Geometry check sheet. Reference: the model listing, model coordinates, mm. Face numbers are marked on the shaded views. A direction names the side the tool comes from. Give positions to 0.01 mm unless a question says otherwise; leave off trailing zeros. Write each loop counter-clockwise with the first axis right and the second up, starting at its lowest first coordinate (ties: lowest second). Pieces come first, ordered by that corner, then holes.
(1) Cross-section at A-A (y = -73.5). Record the boundary of the cut face in (x, z).
(2) Mould release check, pull along Z, two halves, no side actions. Record for the marked faces 5, 6, 7 and 8: +Z half, -Z half, draft (parallel to the pull), parting line (faces both ways), or undercut.
(3) Cross-section at D-D (x = -15). Record the boundary of the cut face in (y, z).
(4) Thickness scan on line 1 along X through (y, z) = (38.5, 31); line 2 along X through (y, z) = (-43.5, 8); line 3 along X through (y, z) = (-17, 9.5). Record the ranges inside material, lowest first.
(5) Depth check by flat-ended pin: P1, Ø8.5, axis at y = -48.5, z = 21.5, coming from the -X side; P2, Ø1, axis at y = 0.5, z = 5.5, coming from the -X side; P3, Ø0.9, axis at y = 38.5, z = 38.5, coming from the -X side. Enter the tip coordinate at first touch or a pass-through.
(6) Cross-section at B-B (x = 38). Record the boundary of the cut face in (y, z).
(7) Tool access check on the marked faces 1, 2, 3 and 4. Record the directions out of +Z, -Z, +X, -X, +Y, -Y that give a thin tool (end or side, any length) a straight path to the whole face; none if there is none.
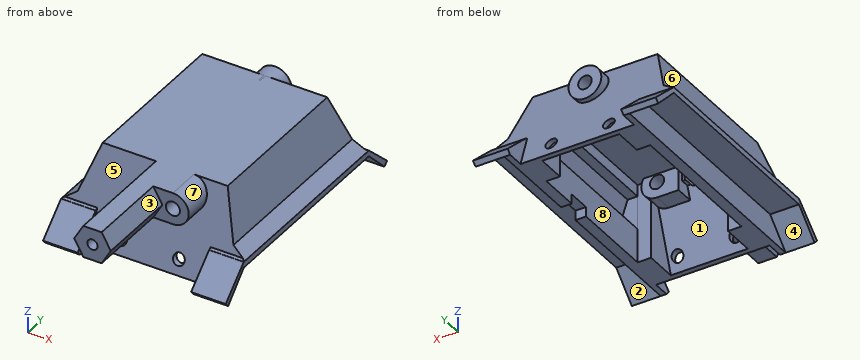
```python
from build123d import *

# Parameters (mm, degrees)
SKETCH_W             = 65
SKETCH_H             = 83
PAD_DEPTH            = 45
SKETCH001_W          = 83
SKETCH001_H          = 32
PAD001_DEPTH         = 15
PAD002_DEPTH         = 15
POCKET_DEPTH         = 403.6691065481
POCKET001_DEPTH      = 500
POCKET001_DEPTH_BACK = 100
PAD003_DEPTH         = 16
SKETCH007_W          = 3
SKETCH007_H          = 135.5960614908
PAD004_DEPTH         = 16
POCKET002_DEPTH      = 414.7315387876
POCKET003_DEPTH      = 5
SKETCH008_W          = 54
SKETCH008_H          = 76
POCKET004_DEPTH      = 35
PAD005_DEPTH         = 65
CHAMFER_SIZE         = 5.3
CHAMFER001_SIZE      = 5.3
CHAMFER002_SIZE      = 0.8999
CHAMFER003_SIZE      = 0.899
CHAMFER004_SIZE      = 0.8999
CHAMFER005_SIZE      = 0.8999
POCKET005_DEPTH      = 80.0010001
POCKET006_DEPTH      = 80.0010001
POCKET007_DEPTH      = 10000
POCKET007_DEPTH_BACK = 100
POCKET008_DEPTH      = 95.001
SKETCH012_W          = 5.5
SKETCH012_H          = 12
POCKET009_DEPTH      = 5
POCKET010_DEPTH      = 20
POCKET010_DEPTH_BACK = 20
POCKET011_DEPTH      = 6
SKETCH014_R          = 8.518625
PAD006_DEPTH         = 13
SKETCH015_R          = 3.5
POCKET012_DEPTH      = 15
SKETCH016_R          = 0.75
POCKET013_DEPTH      = 40
SKETCH018_W          = 5.5
SKETCH018_H          = 12
POCKET014_DEPTH      = 5
POCKET014_FACE131_W  = 12
POCKET014_FACE131_H  = 5.5
PAD007_DEPTH         = 5
POCKET015_DEPTH      = 38.88
POCKET015_DEPTH_BACK = 37
SKETCH020_R          = 3
POCKET016_DEPTH      = 173.1015589479
SKETCH021_R          = 2.7
POCKET017_DEPTH      = 70
SKETCH022_R          = 3.6
PAD008_DEPTH         = 25
SKETCH023_R          = 3.660532
POCKET018_DEPTH      = 25
SKETCH024_W          = 7
SKETCH024_H          = 6.387993
POCKET019_DEPTH      = 40


with BuildPart() as part:
    # Sketch → Pad (new body)
    with BuildSketch(Plane.XY):
        Rectangle(SKETCH_W, SKETCH_H)
    extrude(amount=PAD_DEPTH)

    # Sketch001 (on Face4 of Pad) → Pad001 (join)
    with BuildSketch(Plane(origin=(-32.5, 0, 0), x_dir=(0, -1, 0), z_dir=(-1, 0, 0))):
        with Locations((0, 29)):
            Rectangle(SKETCH001_W, SKETCH001_H)
    pad001 = extrude(amount=PAD001_DEPTH)

    # Mirrored: Pad001 across YZ
    add(pad001.mirror(Plane.YZ))

    # Sketch002 (on Face4 of Mirrored) → Pad002 (join)
    with BuildSketch(Plane.XZ.offset(41.5)):
        Polygon((-47.5, 45), (47.5, 45), (47.5, 13), (32.5, 13), (32.5, 0), (-32.5, 0), (-32.5, 13), (-47.5, 13), align=None)
    pad002 = extrude(amount=PAD002_DEPTH)

    # Mirrored001: Pad002 across XZ
    add(pad002.mirror(Plane.XZ))

    # Sketch003 (on Face13 of Mirrored001) → Pocket (cut, through all)
    with BuildSketch(Plane(origin=(-47.5, 0, 0), x_dir=(0, -1, 0), z_dir=(-1, 0, 0))):
        Polygon((41.5, 45), (56.5, 0), (69.973511, 50.863071), align=None)
    pocket = extrude(amount=-POCKET_DEPTH, mode=Mode.SUBTRACT)

    # Mirrored002: Pocket across XZ
    add(pocket.mirror(Plane.XZ), mode=Mode.SUBTRACT)

    # Sketch004 → Pocket001 (cut, two sides)
    with BuildSketch(Plane.XZ) as pocket001_sk:
        Polygon((-32.5, 45), (-47.5, 0), (-68.972275, 31.059837), (-58.790833, 51.045628), align=None)
    pocket001 = extrude(amount=-POCKET001_DEPTH, mode=Mode.SUBTRACT) + extrude(pocket001_sk.sketch, amount=POCKET001_DEPTH_BACK, mode=Mode.SUBTRACT)

    # Mirrored003: Pocket001 across YZ
    add(pocket001.mirror(Plane.YZ), mode=Mode.SUBTRACT)

    # Sketch006 (on DatumPlane) → Pad003 (join)
    with BuildSketch(Plane(origin=(-47.5, 0, 4), x_dir=(0, -1, 0), z_dir=(-1, 0, 0))):
        Polygon((-68.401131891, -2.9951612268), (-52.1666666667, 12), (52.1666666667, 12), (67.1949295998, -1.7895363668), (65.1666666666, -4), (52.1666666667, 9), (-52.1666666667, 9), (-66.3655953138, -5.1989286472), align=None)
    pad003 = extrude(amount=-PAD003_DEPTH)

    # Sketch007 (on Face8 of Pad003) → Pad004 (join)
    with BuildSketch(Plane(origin=(0, 0, 0), x_dir=(1, 0, 0), z_dir=(0, 0, -1))):
        with Locations((-31, -0.6031011456)):
            Rectangle(SKETCH007_W, SKETCH007_H)
    pad004 = extrude(amount=-PAD004_DEPTH)

    # Pad004 Face41 → Pocket002 (cut, through all)
    with BuildSketch(Plane(origin=(-32.5, 62.9896434829, 11.0016129244), x_dir=(0, 1, 0), z_dir=(-1, 0, 0))):
        Polygon((5.4114884081, -4.9983870756), (5.4114884081, 9.9967741512), (-10.8229768162, -4.9983870756), align=None)
    pocket002 = extrude(amount=-POCKET002_DEPTH, mode=Mode.SUBTRACT)

    # Pocket002 Face27 → Pocket003 (cut)
    with BuildSketch(Plane(origin=(-32.5, -62.1855086221, 11.4034878777), x_dir=(0, 1, 0), z_dir=(-1, 0, 0))):
        Polygon((10.0188419554, -4.5965121223), (-5.0094209777, 9.1930242445), (-5.0094209777, -4.5965121223), align=None)
    pocket003 = extrude(amount=-POCKET003_DEPTH, mode=Mode.SUBTRACT)

    # Mirrored004: Pad003 across YZ
    add(pad003.mirror(Plane.YZ))

    # Mirrored005: Pad004 across YZ
    add(pad004.mirror(Plane.YZ))

    # Mirrored006: Pocket002 across YZ
    add(pocket002.mirror(Plane.YZ), mode=Mode.SUBTRACT)

    # Mirrored007: Pocket003 across YZ
    add(pocket003.mirror(Plane.YZ), mode=Mode.SUBTRACT)

    # Sketch008 (on Face8 of Mirrored007) → Pocket004 (cut)
    with BuildSketch(Plane(origin=(0, 0, 0), x_dir=(1, 0, 0), z_dir=(0, 0, -1))):
        with Locations((0, -0.8994410524)):
            Rectangle(SKETCH008_W, SKETCH008_H)
    extrude(amount=-POCKET004_DEPTH, mode=Mode.SUBTRACT)

    # Sketch009 (on Face24 of Pocket004) → Pad005 (join)
    with BuildSketch(Plane(origin=(0, -37.1005589476, 0), x_dir=(-1, 0, 0), z_dir=(0, 1, 0))):
        Polygon((-4.7576784019, 45), (-9.5153568039, 36.7594592818), (-4.7576784019, 28.5189185635), (4.7576784019, 28.5189185635), (9.5153568039, 36.7594592818), (4.7576784019, 45), align=None)
    extrude(amount=-PAD005_DEPTH)

    # Chamfer
    chamfer_edges = [part.edges().sort_by_distance(p)[0] for p in [
        (42.166667, 0, 16),
    ]]
    chamfer(chamfer_edges, length=CHAMFER_SIZE)

    # Chamfer001
    chamfer001_edges = [part.edges().sort_by_distance(p)[0] for p in [
        (-42.166667, 0, 16),
    ]]
    chamfer(chamfer001_edges, length=CHAMFER001_SIZE)

    # Chamfer002
    chamfer002_edges = [part.edges().sort_by_distance(p)[0] for p in [
        (-44.816667, -51.166667, 16),
        (-37.333333, -51.166667, 16),
        (-32, -51.166667, 16),
        (-30.5, -51.166667, 16),
    ]]
    chamfer(chamfer002_edges, length=CHAMFER002_SIZE)

    # Chamfer003
    chamfer003_edges = [part.edges().sort_by_distance(p)[0] for p in [
        (30.5, -51.166667, 16),
        (32, -51.166667, 16),
        (37.333333, -51.166667, 16),
        (44.816667, -51.166667, 16),
    ]]
    chamfer(chamfer003_edges, length=CHAMFER003_SIZE)

    # Chamfer004
    chamfer004_edges = [part.edges().sort_by_distance(p)[0] for p in [
        (-30.5, 51.166667, 16),
        (-32, 51.166667, 16),
        (-37.333333, 51.166667, 16),
        (-44.816667, 51.166667, 16),
    ]]
    chamfer(chamfer004_edges, length=CHAMFER004_SIZE)

    # Chamfer005
    chamfer005_edges = [part.edges().sort_by_distance(p)[0] for p in [
        (44.816667, 51.166667, 16),
        (37.333333, 51.166667, 16),
        (32, 51.166667, 16),
        (30.5, 51.166667, 16),
    ]]
    chamfer(chamfer005_edges, length=CHAMFER005_SIZE)

    # Chamfer005 Face72 → Pocket005 (cut, through all)
    with BuildSketch(Plane(origin=(-32.5, 68.0917547069, 0.3349462577), x_dir=(0, 1, 0), z_dir=(-1, 0, 0))):
        Polygon((0.3093771841, 0.3349462577), (-0.6187543683, 0.3349462577), (0.3093771841, -0.6698925155), align=None)
    extrude(amount=-POCKET005_DEPTH, mode=Mode.SUBTRACT)

    # Pocket005 Face105 → Pocket006 (cut, through all)
    with BuildSketch(Plane(origin=(-32.5, -66.5188419554, 0.7368212111), x_dir=(0, 1, 0), z_dir=(-1, 0, 0))):
        Polygon((-0.6760876444, -1.4736424221), (1.3521752888, 0.7368212111), (-0.6760876444, 0.7368212111), align=None)
    extrude(amount=-POCKET006_DEPTH, mode=Mode.SUBTRACT)

    # Pocket006 Face73 → Pocket007 (cut, two sides)
    with BuildSketch(Plane(origin=(-31.5, 66.3350874397, -0.3996428824), x_dir=(0, -1, 0), z_dir=(1, 0, 0))) as pocket007_sk:
        Polygon((1.168420773, -0.3996428824), (-0.0305078741, 0.7992857648), (-1.1379128989, -0.3996428824), align=None)
    extrude(amount=-POCKET007_DEPTH, mode=Mode.SUBTRACT)
    extrude(pocket007_sk.sketch, amount=POCKET007_DEPTH_BACK, mode=Mode.SUBTRACT)

    # Sketch011 (on Face39 of Pocket007) → Pocket008 (cut, through all)
    with BuildSketch(Plane.YZ.offset(47.5)):
        Polygon((65.1666666667, 0), (68.818161, 3.6514943333), (70.985268, 1.013342), (68.517616, -0.789946), align=None)
    extrude(amount=-POCKET008_DEPTH, mode=Mode.SUBTRACT)

    # Sketch012 (on Face30 of Pocket008) → Pocket009 (cut)
    with BuildSketch(Plane(origin=(0, 0, 0), x_dir=(1, 0, 0), z_dir=(0, 0, -1))):
        with Locations((-29.75, -11.8994410524)):
            Rectangle(SKETCH012_W, SKETCH012_H)
    extrude(amount=-POCKET009_DEPTH, mode=Mode.SUBTRACT)

    # Sketch013 → Pocket010 (cut, two sides)
    with BuildSketch(Plane.YZ) as pocket010_sk:
        Polygon((-37.1005589476, 35), (-41.46302, 35), (-53.607724, 0), (-37.1005589476, 0), align=None)
    pocket010 = extrude(amount=-POCKET010_DEPTH, mode=Mode.SUBTRACT) + extrude(pocket010_sk.sketch, amount=POCKET010_DEPTH_BACK, mode=Mode.SUBTRACT)

    # Mirrored008: Pocket010 across XZ
    add(pocket010.mirror(Plane.XZ), mode=Mode.SUBTRACT)

    # Mirrored008 Face101 → Pocket011 (cut)
    with BuildSketch(Plane(origin=(0, 0.2373498677, 35), x_dir=(0, -1, 0), z_dir=(0, 0, -1))):
        Polygon((37.3379088153, 27), (-38.6620911847, 27), (-38.6620911847, 20), (-36.86320908, 20), (-36.86320908, -20), (-38.6620911847, -20), (-38.6620911847, -27), (37.3379088153, -27), (37.3379088153, -20), (37.3379088153, -8.4995325139), (37.3379088153, 8.4995325139), (37.3379088153, 20), align=None)
    extrude(amount=-POCKET011_DEPTH, mode=Mode.SUBTRACT)

    # Sketch014 (on Face128 of Pocket011) → Pad006 (join)
    with BuildSketch(Plane.XZ.offset(-37.1005589476)):
        with Locations((0, 36.4884)):
            Circle(SKETCH014_R)
    extrude(amount=-PAD006_DEPTH)

    # Sketch015 (on Face43 of Pad006) → Pocket012 (cut)
    with BuildSketch(Plane(origin=(0, 50.1005589476, 0), x_dir=(-1, 0, 0), z_dir=(0, 1, 0))):
        with Locations((0, 36.4884)):
            Circle(SKETCH015_R)
    extrude(amount=-POCKET012_DEPTH, mode=Mode.SUBTRACT)

    # Sketch016 (on Face67 of Pocket012) → Pocket013 (cut)
    with BuildSketch(Plane.XZ.offset(102.1005589476)):
        with Locations((0, 57.966855919)):
            Circle(SKETCH016_R)
    extrude(amount=-POCKET013_DEPTH, mode=Mode.SUBTRACT)

    # Sketch018 → Pocket014 (cut)
    with BuildSketch(Plane(origin=(0, 0, 0), x_dir=(1, 0, 0), z_dir=(0, 0, -1))):
        with Locations((29.75, -11.8994410524)):
            Rectangle(SKETCH018_W, SKETCH018_H)
    extrude(amount=-POCKET014_DEPTH, mode=Mode.SUBTRACT)

    # Pocket014 Face131 → Pad007 (add)
    with BuildSketch(Plane(origin=(-29.75, 11.8994410524, 5), x_dir=(0, -1, 0), z_dir=(0, 0, -1))):
        Rectangle(POCKET014_FACE131_W, POCKET014_FACE131_H)
    extrude(amount=PAD007_DEPTH)

    # Sketch019 → Pocket015 (cut, two sides)
    with BuildSketch(Plane.XZ) as pocket015_sk:
        Polygon((-29.5, 16.8537200999), (-36.0278850321, 23.381605132), (-32.1550867428, 35), (-27, 35), (-23.389076, 18.833223), align=None)
    pocket015 = extrude(amount=-POCKET015_DEPTH, mode=Mode.SUBTRACT) + extrude(pocket015_sk.sketch, amount=POCKET015_DEPTH_BACK, mode=Mode.SUBTRACT)

    # Mirrored009: Pocket015 across YZ
    add(pocket015.mirror(Plane.YZ), mode=Mode.SUBTRACT)

    # Sketch020 (on DatumPlane) → Pocket016 (cut, through all)
    with BuildSketch(Plane(origin=(0, 71, 34), x_dir=(1, 0, 0), z_dir=(0, 1, 0))):
        with Locations((-15, 26.885509115)):
            Circle(SKETCH020_R)
        with Locations((15, 26.885509115)):
            Circle(SKETCH020_R)
    extrude(amount=-POCKET016_DEPTH, mode=Mode.SUBTRACT)

    # Sketch021 (on Face71 of Pocket016) → Pocket017 (cut)
    with BuildSketch(Plane.XZ.offset(102.1005589476)):
        with Locations((0, 36.7594592818)):
            Circle(SKETCH021_R)
    extrude(amount=-POCKET017_DEPTH, mode=Mode.SUBTRACT)

    # Sketch022 (on DatumPlane) → Pad008 (join)
    with BuildSketch(Plane(origin=(15, -59.1005589476, 12), x_dir=(1, 0, 0), z_dir=(0, -1, 0))):
        with BuildLine():
            ThreePointArc((0, 16.5189185635), (8.2405407182, 24.7594592818), (0, 33))
            Line((0, 33), (-11.193171, 33))
            Line((-11.193171, 33), (-11.193171, 16.5189185635))
            Line((-11.193171, 16.5189185635), (0, 16.5189185635))
        make_face()
        with Locations((0, 24.7594592818)):
            Circle(SKETCH022_R, mode=Mode.SUBTRACT)
    extrude(amount=-PAD008_DEPTH)

    # Sketch023 (on Face73 of Pad008) → Pocket018 (cut)
    with BuildSketch(Plane.XZ.offset(59.1005589476)):
        with Locations((15, 36.7594592818)):
            Circle(SKETCH023_R)
    extrude(amount=-POCKET018_DEPTH, mode=Mode.SUBTRACT)

    # Sketch024 (on Face13 of Pocket018) → Pocket019 (cut)
    with BuildSketch(Plane(origin=(0, 0, 0), x_dir=(1, 0, 0), z_dir=(0, 0, -1))):
        with Locations((0, -38.2690235)):
            Rectangle(SKETCH024_W, SKETCH024_H)
    extrude(amount=-POCKET019_DEPTH, mode=Mode.SUBTRACT)


solid = part.part
```
Reply:
1. outline: (-9.52, 36.76) - (-4.76, 28.52) - (4.76, 28.52) - (9.52, 36.76) - (4.76, 45) - (-4.76, 45) - close; hole circle Ø5.4 at (0, 36.76)
2. face 5: undercut
2. face 6: +Z half
2. face 7: undercut
2. face 8: draft
3. outline: (-56.5, 0) - (-53.61, 0) - (-52.18, 4.11) - (-55.13, 4.11) - close; (-53.13, 10.11) - (-50.1, 10.11) - (-41.46, 35) - (-37.1, 35) - (-37.1, 41) - (37.1, 41) - (37.1, 35) - (41.46, 35) - (50.1, 10.11) - (53.13, 10.11) - (41.5, 45) - (-41.5, 45) - close; (52.18, 4.11) - (53.61, 0) - (56.5, 0) - (55.13, 4.11) - close
4. line 1: x = -37.17 to -33.49, -6.51 to -3.5, 3.5 to 6.51, 33.49 to 37.17
4. line 2: x = -32.5 to -20, 20 to 32.5
4. line 3: x = -32.5 to -27, 27 to 32.5
5. P1: stops at x = -45.73
5. P2: stops at x = -32.5
5. P3: stops at x = -34.82
6. outline: (-67.19, 2.21) - (-65.17, 0) - (-52.17, 13) - (52.17, 13) - (65.17, 0) - (67.24, 2.08) - (52.17, 16) - (52.07, 16) - (50.88, 16.85) - (47, 28.5) - (-47, 28.5) - (-50.88, 16.85) - (-52.07, 16) - (-52.17, 16) - close
7. face 1: -Z
7. face 2: -Z, +X
7. face 3: +Z, +X, -Y
7. face 4: -Z, -X
